Read the model definition and answer for the solid it produces. Units are mm, in the model's axes. A direction names the side the tool comes from. Give positions to 0.01 mm unless a question says otherwise; leave off trailing zeros. Write each loop counter-clockwise with the first axis right and the second up, starting at its lowest first coordinate (ties: lowest second). Pieces come first, ordered by that corner, then holes. Notation, with made-up numbers: (-31, 19.25) - (-22, 19.25) arc R13 ccw to (-22, 32.25) - close; hole circle Ø1 at (28.5, 61). An arc over 180 degrees is marked (long way). Use CSV: the item, a comma, the result in double quotes. Start each with the question number.
from build123d import *

# Parameters (mm, degrees)
SKETCH006_R     = 3.15
PAD002_DEPTH    = 190
SKETCH011_R     = 5
PAD007_DEPTH    = 50
SKETCH010_R     = 5
PAD006_DEPTH    = 50
SKETCH008_R     = 13
PAD004_DEPTH    = 15
SKETCH009_R     = 9
PAD005_DEPTH    = 15
SKETCH013_R     = 6
PAD008_DEPTH    = 26
BOX001_W        = 50
BOX001_H        = 200
BOX001_DEPTH    = 20
SKETCH015_R     = 1.5
POCKET001_DEPTH = 434.247304
SKETCH016_R     = 1.5
POCKET002_DEPTH = 434.247304
SKETCH017_R     = 3
POCKET003_DEPTH = 5
SKETCH018_R     = 3
POCKET004_DEPTH = 5


with BuildPart() as pad002:
    # Sketch006 → Pad002 (new body)
    with BuildSketch(Plane.XZ.offset(80)):
        Circle(SKETCH006_R)
    extrude(amount=-PAD002_DEPTH)


with BuildPart() as pad007:
    # Sketch011 → Pad007 (new body)
    with BuildSketch(Plane.XZ.offset(-75)):
        Circle(SKETCH011_R)
    extrude(amount=PAD007_DEPTH)


with BuildPart() as scassi_perno:
    # Sketch010 → Pad006 (new body)
    with BuildSketch(Plane.XZ.offset(25)):
        Circle(SKETCH010_R)
    extrude(amount=PAD006_DEPTH)

    # Fusion002: union Pad007
    add(pad007.part)


with BuildPart() as scasso_ruota_dentata:
    # Sketch008 → Pad004 (new body)
    with BuildSketch(Plane.XZ.offset(-3)):
        Circle(SKETCH008_R)
    extrude(amount=PAD004_DEPTH)


with BuildPart() as obj1:
    # Sketch009 → Pad005 (new body)
    with BuildSketch(Plane.XZ.offset(-3)):
        with Locations((15.997087, 9e-06)):
            Circle(SKETCH009_R)
    extrude(amount=PAD005_DEPTH)

    # Fusion001: union scasso_ruota_dentata
    add(scasso_ruota_dentata.part)


with BuildPart() as fusion:
    # Sketch013 → Pad008 (new body)
    with BuildSketch(Plane.XZ.offset(11)):
        with Locations((16.059561, 9e-06)):
            Circle(SKETCH013_R)
    extrude(amount=PAD008_DEPTH)

    # Fusion005: union scassi_perno, obj1
    add(scassi_perno.part)
    add(obj1.part)

    # Fusion: union Pad002
    add(pad002.part)


with BuildPart() as obj2:
    # Box001 → Box001 (new body)
    with BuildSketch(Plane(origin=(-20, -100, -21), x_dir=(1, 0, 0), z_dir=(0, 0, 1))):
        with Locations((25, 100)):
            Rectangle(BOX001_W, BOX001_H)
    extrude(amount=BOX001_DEPTH)

    # Cut001: cut Fusion
    add(fusion.part, mode=Mode.SUBTRACT)

    # Sketch015 → Pocket001 (cut, through all)
    with BuildSketch(Plane(origin=(0, 0, -21), x_dir=(1, 0, 0), z_dir=(0, 0, -1))):
        with Locations((23, 90)):
            Circle(SKETCH015_R)
    pocket001 = extrude(amount=-POCKET001_DEPTH, mode=Mode.SUBTRACT)

    # Mirrored: Pocket001 across Sketch015 H_Axis
    add(pocket001.mirror(Plane(origin=(0, 0, -21), x_dir=(0, 0, -1), z_dir=(0, -1, 0))), mode=Mode.SUBTRACT)

    # Sketch016 → Pocket002 (cut, through all)
    with BuildSketch(Plane(origin=(0, 0, -21), x_dir=(1, 0, 0), z_dir=(0, 0, -1))):
        with Locations((-12, 90)):
            Circle(SKETCH016_R)
    pocket002 = extrude(amount=-POCKET002_DEPTH, mode=Mode.SUBTRACT)

    # Mirrored001: Pocket002 across Sketch016 H_Axis
    add(pocket002.mirror(Plane(origin=(0, 0, -21), x_dir=(0, 0, -1), z_dir=(0, -1, 0))), mode=Mode.SUBTRACT)

    # Sketch017 → Pocket003 (cut)
    with BuildSketch(Plane(origin=(0, 0, -21), x_dir=(1, 0, 0), z_dir=(0, 0, -1))):
        with Locations((23, 90)):
            Circle(SKETCH017_R)
    pocket003 = extrude(amount=-POCKET003_DEPTH, mode=Mode.SUBTRACT)

    # Mirrored002: Pocket003 across Sketch017 H_Axis
    add(pocket003.mirror(Plane(origin=(0, 0, -21), x_dir=(0, 0, -1), z_dir=(0, -1, 0))), mode=Mode.SUBTRACT)

    # Sketch018 → Pocket004 (cut)
    with BuildSketch(Plane(origin=(0, 0, -21), x_dir=(1, 0, 0), z_dir=(0, 0, -1))):
        with Locations((-12, 90)):
            Circle(SKETCH018_R)
    pocket004 = extrude(amount=-POCKET004_DEPTH, mode=Mode.SUBTRACT)

    # Mirrored003: Pocket004 across Sketch018 H_Axis
    add(pocket004.mirror(Plane(origin=(0, 0, -21), x_dir=(0, 0, -1), z_dir=(0, -1, 0))), mode=Mode.SUBTRACT)


solid = obj2.part
(1) For a pull along Y with two mould halves and no side action, classify faces 6 (the face through (24.3, 88.7, -16)), 7 (the face through (-0.06, 87.32, -3.15)), 8 (the face through (5, -100, -11)) as pulls with the +Y half, pulls with the -Y half, needs draft (parallel to the pull), parting line crosses it, or undercut.
(2) The part is cut by section B-B on y = 52. Write down the section's boundary in (x, z), plus the area to 3 significant figures.
(3) The part is cut by section A-A on z = -11. Write down the section's boundary in (x, y), plus the area to 3 significant figures.
(4) Which of the six approach directions +Z, -Z, +X, -X, +Y, -Y give full straight-line access (tool end or side, diameter ignored) to faces 1 (the face through (-0.06, 13.85, -3.15)), 2 (the face through (5, -21, -1)), 3 (the face through (22.35, 87.07, -18.54)), 4 (the face through (16, -24, -6)), 5 (the face through (5, 1, -21))?
(5) The part is cut by section C-C on x = 14.5. Write down the section's boundary in (y, z).
(6) Consider probe 1 along Y at (x, z) = (23, -7); probe 2 along X at (y, z) = (90, -11.75); probe 3 along X at (y, z) = (90, -17). Determine where each line is inside the solid, lowest interval first.
(7) Given P1, Ø1.8, axis at x = -12.5, y = -88.5, coming from the -Z side, flat-ended and moving along its own axis, determine where the tip first touches the part or whether it passes through.
Reported:
1,face 6,"undercut"
1,face 7,"needs draft"
1,face 8,"pulls with the -Y half"
2,outline,"(-20, -21) - (30, -21) - (30, -1) - (4.9, -1) arc R5 cw to (-4.9, -1) - (-20, -1) - close"
2,area,"971 mm²"
3,outline,"(-20, -100) - (30, -100) - (30, 100) - (-20, 100) - close; hole circle Ø3 at (-12, -90); hole circle Ø3 at (-12, 90); hole (-6.93, -12) - (6.93, -12) - (6.93, 3) - (-6.93, 3) - close; hole circle Ø3 at (23, -90); hole circle Ø3 at (23, 90)"
3,area,"9,760 mm²"
4,face 1,"+Z, +Y"
4,face 2,"+Z, +X, -X, +Y, -Y"
4,face 3,"-Z"
4,face 4,"+Z"
4,face 5,"-Z, +X, -X, +Y, -Y"
5,outline,"(-100, -21) - (100, -21) - (100, -1) - (3, -1) - (3, -8.87) - (-12, -8.87) - (-12, -5.79) - (-37, -5.79) - (-37, -1) - (-100, -1) - close"
6,probe 1,"-100 to -91.5, -88.5 to 88.5, 91.5 to 100"
6,probe 2,"-20 to -13.5, -10.5 to 21.5, 24.5 to 30"
6,probe 3,"-20 to -15, -9 to 20, 26 to 30"
7,P1,"z = -16"
